Autodesk Inventor part; units mm, degrees
ref_plane "Work Plane1" through (39.6875, -5.6924, 0) normal (-0.0676, 0.9977, 0) x (-0.9977, -0.0676, 0)
ref_plane "Work Plane2" through (0, -14.7343, 0) normal (-0.3713, 0.9285, 0) x (-0.9285, -0.3713, 0)
ref_plane "YZ Plane" through (0, 0, 0) normal (1, 0, 0) x (0, 1, 0)
sketch "Sketch1" plane through (0, 0, 0) normal (0, 0, 1) x (1, 0, 0)
  arc A0 (10.3242, -27.9992) -> (11.7654, -28.1173) centre (11.0677, -27.7785) ccw
  line L0 (11.7654, -28.1173) -> (12.9919, -27.5665)
  arc A1 (12.9919, -27.5665) -> (34.2886, -13.9193) centre (16.4917, -9.5875) ccw
  arc A2 (10.3242, -27.9992) -> (0, -14.7343) centre (-11.7995, -34.5682) ccw
  arc A3 (5.5815, -12.6488) -> (14.136, -24.6939) centre (18.1207, -12.8036) ccw
  arc A4 (32.6339, -13.5274) -> (32.5628, -6.3713) centre (17.9412, -10.0948) ccw
  arc A5 (39.6875, -5.6924) -> (34.2886, -13.9193) centre (48.5431, -17.3889) ccw
  arc A6 (5.5815, -12.6488) -> (0, -14.7343) centre (48.5171, -136.0683) ccw
  arc A7 (39.6875, -5.6924) -> (32.5628, -6.3713) centre (48.5171, -136.0683) ccw
  arc A8 (14.136, -24.6939) -> (32.6339, -13.5274) centre (17.9429, -10.0956) ccw
  point P0 (0, 0)
extrude "Extrusion1" add sketch "Sketch1" along normal blind 8.98
ref_plane "Work Plane1" through (39.6875, -5.6924, 0) normal (-0.0676, 0.9977, 0) x (-0.9977, -0.0676, 0)
sketch "Sketch2" plane through (39.6875, -5.6924, 0) normal (-0.0676, 0.9977, 0) x (-0.9977, -0.0676, 0)
  circle A0 centre (2.81, 4.525) radius 1
  line L0 (7.1542, 0) -> (0, 0)
  line L1 (0, 0) -> (0, 8.98)
  point P0 (39.2122, 0)
  dimension "d2" = 2
  dimension "d15" = 4.525
  dimension "d16" = 2.81
extrude "Extrusion2" cut sketch "Sketch2" against normal through all
thread "Thread1"
ref_plane "Work Plane2" through (0, -14.7343, 0) normal (-0.3713, 0.9285, 0) x (-0.9285, -0.3713, 0)
sketch "Sketch3" plane through (0, -14.7343, 0) normal (-0.3713, 0.9285, 0) x (-0.9285, -0.3713, 0)
  circle A0 centre (-3, 4.455) radius 1
  line L0 (0, 0) -> (0, 8.98)
  line L1 (0, 8.98) -> (-5.9568, 8.98)
  line L2 (0, 0) -> (-5.9568, 0)
  point P0 (-5.4706, 0)
  dimension "d7" = 2
  dimension "d12" = 3
  dimension "d13" = 4.525
  dimension "d14" = 8.98
extrude "Extrusion3" cut sketch "Sketch3" against normal through all
thread "Thread2"
properties material "Liga de Nickel-Copper 400"
Could you check a few things on this model? Use its own coordinates, in mm. A direction names the side the tool comes from. Coordinates: 2 decimals unless noted, no trailing zeros. Order: outer loops, then holes, each group sorted by start corner. A loop starts at its lowest first (then second) coordinate and runs counter-clockwise, first axis right, second up. Notation, with made-up numbers: (-39, 70.5) -> (6, 70.5) arc R30 ccw to (6, 100.5) -> close; hole circle Ø7 at (58.25, -39). An arc over 180 degrees is marked (long way). One line per item, written item: value. Start each with the question number.
1) We'd pull the mould along Z, two halves only. Please class faces 3 (the cylindrical face through (26.54, -24.9, 4.43)), 4 (the flat face through (23, -25, 8.98)), 5 (the flat face through (23, -25, 0)), 6 (the cylindrical face through (4.875, -16.155, 4.499)): +Z half, -Z half, draft (parallel to the pull), parting line (faces both ways), or undercut.
2) I'm going to push flat-ended pins straight in: pin 1 (2 mm diameter, centred on x = 30.5, z = 4.5, fed in from +Y); pin 2 (1.5 mm diameter, centred on x = 22.5, z = 6, fed in from -Y); pin 3 (2 mm diameter, centred on x = 21, z = 3, fed in from +Y). Where does each tip first touch, or does it pass through?
3) Imagine slicing it at D-D on y = -26.25. List the corners of the cut face in (x, z) for me.
4) Which directions (+Z, -Z, +X, -X, +Y, -Y) give clear straight access to the entire face, cutting with the end or side of a thin tool? Please do faces 1 (the cylindrical face through (36.03, -7.34, 4.83)), 2 (the flat face through (12.37, -27.846, 4.427)).
5) Imagine slicing it at B-B on y = -22.25. List the corners of the cut face in (x, z) for me.
6) If I drill on L1, parallel to X at y = -19.75, z = 3; L2, parallel to X at y = -25.25, z = 1.5; L3, parallel to X at y = -7, z = 1.5, over which ranges is the centre line in solid material (lowest first)? Write a range as [from, to].
7) Imagine slicing it at A-A on z = 6.25. List the corners of the cut face in (x, y) for me, plus the area to 3 significant figures.
8) Imagine slicing it at C-C on x = 21.5. List the corners of the cut face in (y, z) for me.
Answer list:
1. face 3: draft
1. face 4: +Z half
1. face 5: -Z half
1. face 6: undercut
2. pin 1: stops at y = -16.71
2. pin 2: stops at y = -27.13
2. pin 3: stops at y = -24.63
3. outline: (9.73, 0) -> (24.1, 0) -> (24.1, 8.98) -> (9.73, 8.98) -> close
4. face 1: none
4. face 2: +Z, -Z, -Y
5. outline: (7.72, 0) -> (9.87, 0) -> (9.87, 8.98) -> (7.72, 8.98) -> close; (26.88, 0) -> (29.73, 0) -> (29.73, 8.98) -> (26.88, 8.98) -> close
6. L1: x = [5.89, 7.68], [29.54, 31.73]
6. L2: x = [9.31, 25.99]
6. L3: x = [32.71, 38.18]
7. outline: (0, -14.73) arc R23.08 cw to (10.32, -28) arc R0.78 ccw to (11.77, -28.12) -> (12.99, -27.57) arc R18.32 ccw to (34.29, -13.92) arc R14.67 cw to (39.69, -5.69) arc R130.75 ccw to (32.56, -6.37) arc R15.09 cw to (32.63, -13.53) arc R15.09 cw to (14.14, -24.69) arc R12.54 cw to (5.58, -12.65) arc R130.75 ccw to start
7. area: 129 mm2
8. outline: (-27.21, 0) -> (-24.76, 0) -> (-24.76, 8.98) -> (-27.21, 8.98) -> close
